Design review of the part built by this model. Coordinates are the model's own, in mm. Face numbers are marked on the shaded views. A direction names the side the tool comes from. Coordinates: 2 decimals unless noted, no trailing zeros. Write each loop counter-clockwise with the first axis right and the second up, starting at its lowest first coordinate (ties: lowest second). Pieces come first, ordered by that corner, then holes. Notation, with made-up numbers: M -30,-27.5 L 4,-27.5 A23 cw 4,10.5 Z; hole C 19,-32.75 d5. An arc over 180 degrees is marked long. Write item = value, one per line.
```python
from build123d import *

# Parameters (mm, degrees)
BOSS_EXTRUDE1_DEPTH = 8
CUT_EXTRUDE1_DEPTH  = 10
SKETCH3_R           = 1.75
CUT_EXTRUDE2_DEPTH  = 10
FILLET1_R           = 10
BOSS_EXTRUDE2_DEPTH = 8
CHAMFER1_SIZE       = 3
SKETCH5_R           = 3.1
CUT_EXTRUDE3_DEPTH  = 4
BOSS_EXTRUDE3_DEPTH = 8
SKETCH9_R           = 4
BOSS_EXTRUDE5_DEPTH = 14
SKETCH10_R          = 1.75
CUT_EXTRUDE4_DEPTH  = 37
FILLET4_R           = 1
CUT_EXTRUDE5_DEPTH  = 10
FILLET9_R           = 6
FILLET10_R          = 6
SKETCH13_R          = 1.948575194
SKETCH13_R_2        = 1.8
CUT_EXTRUDE7_DEPTH  = 22


with BuildPart() as part:
    # Sketch1 → Boss-Extrude1 (new body)
    with BuildSketch(Plane.XY):
        Polygon((30.83321951, 51.480464718), (-29.16678049, 52.442583736), (-60, 0.962119017), (-30.83321951, -51.480464718), (29.16678049, -52.442583736), (60, -0.962119017), align=None)
    extrude(amount=BOSS_EXTRUDE1_DEPTH)

    # Sketch2 → Cut-Extrude1 (cut)
    with BuildSketch(Plane.XY.offset(8)):
        Polygon((-21.388972359, 38.45789474), (-44, 0.705553946), (-22.611027641, -37.752340793), (21.388972359, -38.45789474), (44, -0.705553946), (22.611027641, 37.752340793), align=None)
    extrude(amount=-CUT_EXTRUDE1_DEPTH, mode=Mode.SUBTRACT)

    # Sketch3 → Cut-Extrude2 (cut)
    with BuildSketch(Plane(origin=(0, 0, 0), x_dir=(-1, 0, 0), z_dir=(0, 0, -1))):
        with Locations((-9.276605543, -45.192747573)):
            Circle(SKETCH3_R)
        with Locations(Location((10.720823639, -44.872082458, 0), (0, 0, 180))):
            Circle(SKETCH3_R)
        with Locations((-34.499764694, 30.630149848)):
            Circle(SKETCH3_R)
        with Locations(Location((-44.220775149, 13.151535608, 0), (0, 0, 180))):
            Circle(SKETCH3_R)
        with Locations((43.776370237, 14.562597726)):
            Circle(SKETCH3_R)
        with Locations(Location((33.49995151, 31.72054685, 0), (0, 0, 180))):
            Circle(SKETCH3_R)
    extrude(amount=-CUT_EXTRUDE2_DEPTH, mode=Mode.SUBTRACT)

    # Fillet1
    fillet1_edges = [part.edges().sort_by_distance(p)[0] for p in [
        (60, -0.962119017, 4),
        (29.16678049, -52.442583736, 4),
        (-30.83321951, -51.480464718, 4),
        (-60, 0.962119017, 4),
        (-29.16678049, 52.442583736, 4),
        (30.83321951, 51.480464718, 4),
        (-21.388972359, 38.45789474, 4),
        (22.611027641, 37.752340793, 4),
        (44, -0.705553946, 4),
        (21.388972359, -38.45789474, 4),
        (-22.611027641, -37.752340793, 4),
        (-44, 0.705553946, 4),
    ]]
    fillet(fillet1_edges, radius=FILLET1_R)

    # Sketch4 → Boss-Extrude2 (add)
    with BuildSketch(Plane(origin=(0, 0, 0), x_dir=(-1, 0, 0), z_dir=(0, 0, -1))):
        Polygon((-30.389210684, 23.766977696), (36.221816957, -13.279809152), (30.389210684, -23.766977696), (-36.221816957, 13.279809152), align=None)
    extrude(amount=-BOSS_EXTRUDE2_DEPTH)

    # Chamfer1
    chamfer1_edges = [part.edges().sort_by_distance(p)[0] for p in [
        (-30.389210684, -23.766977696, 4),
        (-36.221816957, -13.279809152, 4),
        (30.389210684, 23.766977696, 4),
        (36.221816957, 13.279809152, 4),
    ]]
    chamfer(chamfer1_edges, length=CHAMFER1_SIZE)

    # Sketch5 → Cut-Extrude3 (cut)
    with BuildSketch(Plane(origin=(0, 0, 0), x_dir=(-1, 0, 0), z_dir=(0, 0, -1))):
        with Locations((43.776370237, 14.562597726)):
            Circle(SKETCH5_R)
        with Locations((33.49995151, 31.72054685)):
            Circle(SKETCH5_R)
        with Locations((-9.276605543, -45.192747573)):
            Circle(SKETCH5_R)
        with Locations((10.720823639, -44.872082458)):
            Circle(SKETCH5_R)
        with Locations((-34.499764694, 30.630149848)):
            Circle(SKETCH5_R)
        with Locations((-44.220775149, 13.151535608)):
            Circle(SKETCH5_R)
    extrude(amount=-CUT_EXTRUDE3_DEPTH, mode=Mode.SUBTRACT)

    # Sketch7 → Boss-Extrude3 (add)
    with BuildSketch(Plane(origin=(0, 0, 0), x_dir=(-1, 0, 0), z_dir=(0, 0, -1))):
        Polygon((-1.453350423, 7.673836886), (20.4189231, 47.000718924), (29.15823022, 42.140213697), (7.285956696, 2.813331658), align=None)
        Polygon((1.453350423, -7.673836886), (-20.4189231, -47.000718924), (-29.15823022, -42.140213697), (-7.285956696, -2.813331658), align=None)
    extrude(amount=-BOSS_EXTRUDE3_DEPTH)

    # Sketch9 → Boss-Extrude5 (add)
    with BuildSketch(Plane(origin=(0, 0, 0), x_dir=(-1, 0, 0), z_dir=(0, 0, -1))):
        with Locations(Location((39.520199599, -21.478309331, 0), (0, 0, 180))):
            Circle(SKETCH9_R)
        with Locations(Location((-38.471532181, -23.301561321, 0), (0, 0, 180))):
            Circle(SKETCH9_R)
        with Locations(Location((-1.054648832, 45.15288568, 0), (0, 0, 180))):
            Circle(SKETCH9_R)
    extrude(amount=BOSS_EXTRUDE5_DEPTH)

    # Sketch10 → Cut-Extrude4 (cut)
    with BuildSketch(Plane(origin=(0, 0, -14), x_dir=(-1, 0, 0), z_dir=(0, 0, -1))):
        with Locations((-38.471532181, -23.301561321)):
            Circle(SKETCH10_R)
        with Locations((-0.943977962, 44.968104852)):
            Circle(SKETCH10_R)
        with Locations((39.415510143, -21.66654353)):
            Circle(SKETCH10_R)
    extrude(amount=-CUT_EXTRUDE4_DEPTH, mode=Mode.SUBTRACT)

    # Fillet4
    fillet4_edges = [part.edges().sort_by_distance(p)[0] for p in [
        (-43.520199599, -21.478309331, 0),
        (34.471532181, -23.301561321, 0),
        (-2.945351168, 45.15288568, 0),
    ]]
    fillet(fillet4_edges, radius=FILLET4_R)

    # Sketch11 → Cut-Extrude5 (cut)
    with BuildSketch(Plane(origin=(0, 0, 0), x_dir=(-1, 0, 0), z_dir=(0, 0, -1))):
        with BuildLine():
            Line((-7.524180813, 7.045332007), (9.954433427, -2.675678448))
            ThreePointArc((9.954433427, -2.675678448), (10.9241339, -6.075631534), (7.524180813, -7.045332007))
            Line((7.524180813, -7.045332007), (-9.954433427, 2.675678448))
            ThreePointArc((-9.954433427, 2.675678448), (-10.9241339, 6.075631534), (-7.524180813, 7.045332007))
        make_face()
    extrude(amount=-CUT_EXTRUDE5_DEPTH, mode=Mode.SUBTRACT)

    # Fillet9
    fillet9_edges = [part.edges().sort_by_distance(p)[0] for p in [
        (24.355518918, -33.504821467, 4),
        (15.616211798, -38.365326694, 4),
        (-24.355518918, 33.504821467, 4),
        (-15.616211798, 38.365326694, 4),
    ]]
    fillet(fillet9_edges, radius=FILLET9_R)

    # Fillet10
    fillet10_edges = [part.edges().sort_by_distance(p)[0] for p in [
        (1.453350423, 7.673836886, 4),
        (-7.285956696, 2.813331658, 4),
        (-1.453350423, -7.673836886, 4),
        (7.285956696, -2.813331658, 4),
    ]]
    fillet(fillet10_edges, radius=FILLET10_R)

    # Sketch13 → Cut-Extrude7 (cut)
    with BuildSketch(Plane(origin=(0, 0, 0), x_dir=(-1, 0, 0), z_dir=(0, 0, -1))):
        with Locations((-14.094687316, -25.342592065)):
            Circle(SKETCH13_R)
        with Locations((14.096243004, 25.34538923)):
            Circle(SKETCH13_R_2)
    extrude(amount=-CUT_EXTRUDE7_DEPTH, mode=Mode.SUBTRACT)


solid = part.part
```
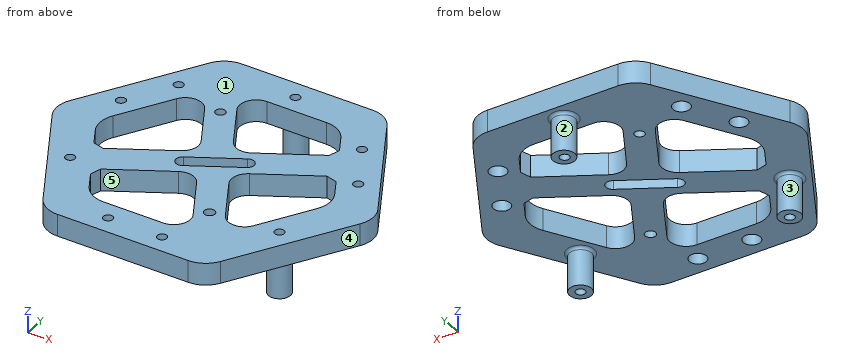
Q1. For P1, Ø5, axis at x = 44.22, y = 13.15, coming from the -Z side; P2, Ø3, axis at x = -10.72, y = -44.87, coming from the -Z side (3 decimals); P3, Ø5, axis at x = 14.09, y = -25.34, coming from the -Z side; P4, Ø4, axis at y = -13.5, z = 2.5, coming from the -X side, all flat-tipped, find the tip position at first contact; note any pin that passes through.
Check result:
P1 = 4
P2 = through
P3 = 0
P4 = -53.07
Q2. Machinability: for the marked faces 4 and 5, which of the approach directions +Z, -Z, +X, -X, +Y, -Y give a long, thin tool a straight path to every point of the face, cutting with its end or side? Answer none if there is none.
Check result:
face_4 = +Z, -Z, +X, -Y
face_5 = +Z, -Z
Q3. Wall thickness on line 1 (Y direction, x = -20, z = 2); line 2 (Y direction, x = -6.5, z = 0.25); line 3 (Y direction, x = 7.5, z = 3.5): over which ranges is each line inside the solid? List them lowest first.
Check result:
line_1 = -51.65 to -37.28, -17.99 to -4.26, 25.42 to 52.3
line_2 = -51.87 to -38.01, -10.49 to -6.48, -0.75 to 21.97, 38.08 to 52.08
line_3 = -52.1 to -47.73, -42.65 to -37.79, -23.77 to 1.31, 7.03 to 11.04, 37.99 to 51.85
Q4. Consider section A-A, the plane z = -10. State the section outline as (x, y) points, and give its area (3 significant figures).
Check result:
outline = C -39.52,-21.48 d8; C 1.05,45.15 d8; C 38.47,-23.3 d8; hole C -39.42,-21.67 d3.5; hole C 0.94,44.97 d3.5; hole C 38.47,-23.3 d3.5
area = 122 mm²
Q5. The part is to be moulded in two halves that separate along X. For the marked faces 1, 2 and 3, say which applies: +X half, -X half, draft (parallel to the pull), parting line (faces both ways), or undercut.
Check result:
face_1 = draft
face_2 = parting line
face_3 = undercut
Q6. Consider section B-B, the plane y = -36.5. State the section outline as (x, z) points.
Check result:
outline = M -39.16,0 L -21.69,0 L -21.69,8 L -39.16,8 Z; M 9.51,0 L 38.72,0 L 38.72,8 L 9.51,8 Z
